```python
from build123d import *

# Parameters (mm, degrees)
SKETCH_1_R               = 1.65
EXTRUDE_3_DEPTH          = 3
SKETCH_3_W               = 54
SKETCH_3_H               = 42
SKETCH_3_W_2             = 48
SKETCH_3_H_2             = 36
EXTRUDE_4_DEPTH          = 8
CUT_EXTRUDE_1_DEPTH      = 1
CUT_EXTRUDE_1_DEPTH_BACK = 43
SKETCH_5_W               = 8
SKETCH_5_H               = 14
CUT_EXTRUDE_2_DEPTH      = 61


with BuildPart() as part:
    # 草图1 → 凸台-拉伸3 (new body)
    with BuildSketch(Plane.XY):
        Polygon((0, 21), (-30, 21), (-33, 21), (-33, -21), (33, -21), (33, 21), align=None)
        with Locations((-30, -11.316768896)):
            Circle(SKETCH_1_R, mode=Mode.SUBTRACT)
        with BuildLine():
            ThreePointArc((-30, 13.033231104), (-31.65, 14.683231104), (-30, 16.333231104))
            ThreePointArc((-30, 16.333231104), (-28.35, 14.683231104), (-30, 13.033231104))
        make_face(mode=Mode.SUBTRACT)
        with Locations((30, 14.683231104)):
            Circle(SKETCH_1_R, mode=Mode.SUBTRACT)
        with Locations((30, -11.316768896)):
            Circle(SKETCH_1_R, mode=Mode.SUBTRACT)
    extrude(amount=EXTRUDE_3_DEPTH)

    # 草图3 → 凸台-拉伸4 (add)
    with BuildSketch(Plane.XY.offset(3)):
        Rectangle(SKETCH_3_W, SKETCH_3_H)
        Rectangle(SKETCH_3_W_2, SKETCH_3_H_2, mode=Mode.SUBTRACT)
    extrude(amount=EXTRUDE_4_DEPTH)

    # 草图4 → 切除-拉伸1 (cut, two sides)
    with BuildSketch(Plane.XZ.offset(21)) as cut_extrude_1_sk:
        Polygon((-10, 109.769364085), (-10, 11), (-10, 3), (10, 3), (10, 11), (10, 109.769364085), (10, 307.308092254), (-10, 307.308092254), align=None)
    extrude(amount=CUT_EXTRUDE_1_DEPTH, mode=Mode.SUBTRACT)
    extrude(cut_extrude_1_sk.sketch, amount=-CUT_EXTRUDE_1_DEPTH_BACK, mode=Mode.SUBTRACT)

    # 草图5 → 切除-拉伸2 (cut, through all)
    with BuildSketch(Plane.ZY.offset(27)):
        with Locations((7, 0)):
            Rectangle(SKETCH_5_W, SKETCH_5_H)
    extrude(amount=-CUT_EXTRUDE_2_DEPTH, mode=Mode.SUBTRACT)


solid = part.part
```
Build history of the part. All positions in model axes, mm. A direction names the side the tool comes from. Give positions to 0.01 mm unless a question says otherwise; leave off trailing zeros. Loops run counter-clockwise (first coordinate to the right, second up) from the corner with the lowest first, then second, coordinate; pieces in that order, holes last. Notation, with made-up numbers: (-1, 74) -> (54, 74) arc R24 cw to (54, 104) -> close; hole circle Ø7 at (14.5, 41). An arc over 180 degrees is marked (long way). One line per question, with ' | ' between items. Start each with the question number.
1) Pin check, flat tips, straight feed: pin 1 (4.5 mm diameter, centred on x = 30, y = -11.32, fed in from +Z); pin 2 (3 mm diameter, centred on x = 12.5, y = -1.5, fed in from -Z); pin 3 (1.5 mm diameter, centred on y = -19.5, z = 5.5, fed in from -X); pin 4 (4 mm diameter, centred on y = 14, z = 8, fed in from +X). Stop position of each tip, or through.
2) 3-axis set-ups, long thin cutter, end or side, ignore diameter. For faces 4 (the flat face through (-10, 19, 7)), 5 (the flat face through (-26, -7, 7)), 6 (the flat face through (27, -14, 7)), 7 (the flat face through (24, -13, 7)): which of +Z, -Z, +X, -X, +Y, -Y reach the whole face in a straight line?
3) Two-plate mould, pull along Y, no slides. Class faces 1 (the flat face through (0, -21, 2)), 2 (the flat face through (25, -7, 7)), 3 (the flat face through (22, -19, 11)): released by +Y, released by -Y, zero draft, split by the parting line, or undercut.
4) Cut at D-D (y = -3.5). Give the cut face in (x, z).
5) Probe L1, parallel to Y at x = 30, z = 2.25; L2, parallel to X at y = -8, z = 6.5; L3, parallel to Y at x = 28.5, z = 2.75. List the from-to ranges inside material, lowest first.
6) Cut at B-B (x = 30). Give the cut face in (y, z).
7) Cut at A-A (z = 7). Give the cut face in (x, y).
8) Cut at C-C (x = -11). Give the cut face in (y, z), plus the area to 3 significant figures.
Return value:
1) pin 1: z = 3 | pin 2: z = 0 | pin 3: x = -27 | pin 4: x = 27
2) face 4: +Z, +Y, -Y | face 5: +Z, +X, -X | face 6: +Z, +X, +Y, -Y | face 7: +Z
3) face 1: released by -Y | face 2: undercut | face 3: zero draft
4) outline: (-33, 0) -> (33, 0) -> (33, 3) -> (-33, 3) -> close
5) L1: -21 to -12.97, -9.67 to 13.03, 16.33 to 21 | L2: -27 to -24, 24 to 27 | L3: -21 to -12, -10.63 to 14, 15.37 to 21
6) outline: (-21, 0) -> (-12.97, 0) -> (-12.97, 3) -> (-21, 3) -> close; (-9.67, 0) -> (13.03, 0) -> (13.03, 3) -> (-9.67, 3) -> close; (16.33, 0) -> (21, 0) -> (21, 3) -> (16.33, 3) -> close
7) outline: (-27, -21) -> (-10, -21) -> (-10, -18) -> (-24, -18) -> (-24, -7) -> (-27, -7) -> close; (-27, 7) -> (-24, 7) -> (-24, 18) -> (-10, 18) -> (-10, 21) -> (-27, 21) -> close; (10, -21) -> (27, -21) -> (27, -7) -> (24, -7) -> (24, -18) -> (10, -18) -> close; (10, 18) -> (24, 18) -> (24, 7) -> (27, 7) -> (27, 21) -> (10, 21) -> close
8) outline: (-21, 0) -> (21, 0) -> (21, 11) -> (18, 11) -> (18, 3) -> (-18, 3) -> (-18, 11) -> (-21, 11) -> close | area: 174 mm^2
